Build history of the part. All positions in model axes, mm. A direction names the side the tool comes from. Give positions to 0.01 mm unless a question says otherwise; leave off trailing zeros. Order: outer loops, then holes, each group sorted by start corner. A loop starts at its lowest first (then second) coordinate and runs counter-clockwise, first axis right, second up. Notation, with made-up numbers: (23.5, -37.5) - (47.5, -37.5) arc R10 ccw to (47.5, -26.5) - close; hole circle Ø6 at (31, 3.25). An arc over 180 degrees is marked (long way). Answer in a Markdown table with one row per item.
```python
from build123d import *

# Parameters (mm, degrees)
F0_W     = 76.2
F0_H     = 76.2
F1_DEPTH = 76.2
F2_W     = 25.4
F2_H     = 25.4
F3_DEPTH = 12.7
F5_D     = 25.4
F6_R     = 15.048086
F7_DEPTH = 12.7


with BuildPart() as f1:
    # F0 (on Front) → F1 (new body)
    with BuildSketch(Plane.XZ):
        with Locations((5.308721, 14.755955)):
            Rectangle(F0_W, F0_H)
    extrude(amount=F1_DEPTH)

    # F2 (on face) → F3 (join)
    with BuildSketch(Plane.XZ.offset(76.2)):
        with Locations((5.308721, 14.755955)):
            Rectangle(F2_W, F2_H)
    extrude(amount=F3_DEPTH)

    # F5 (through all)
    with Locations(Plane.XY.offset(52.855955)):
        with Locations((0, -38.1)):
            Hole(F5_D / 2)

    # F6 (on face) → F7 (join)
    with BuildSketch(Plane.YZ.offset(43.408721)):
        with Locations((-40.448086, 17.104041)):
            Circle(F6_R)
    extrude(amount=F7_DEPTH)


solid = f1.part
```
1. Drop flat-ended pins along their axis: P1, Ø6.5, axis at x = 6.5, y = -81.5, coming from the +Z side; P2, Ø10, axis at y = -85, z = 10.5, coming from the +X side; P3, Ø6, axis at x = 40, z = 18.5, coming from the -Y side. Give the stop position or say it passes through.
Check result:
| item | result |
|---|---|
| P1 | stops at z = 27.46 |
| P2 | stops at x = 18.01 |
| P3 | stops at y = -76.2 |
2. Cut at B-B on y = -38.1. Write the cut outline in (x, z), and give its area (3 significant figures).
Check result:
| item | result |
|---|---|
| outline | (-32.79, -23.34) - (-12.7, -23.34) - (-12.7, 52.86) - (-32.79, 52.86) - close; (12.7, -23.34) - (43.41, -23.34) - (43.41, 2.24) - (56.11, 2.24) - (56.11, 31.97) - (43.41, 31.97) - (43.41, 52.86) - (12.7, 52.86) - close |
| area | 4,250 mm² |
3. Probe line 1 (Y direction, x = 0, z = 7); line 2 (Y direction, x = 0, z = -6); line 3 (X direction, y = -38, z = -4). List the from-to ranges inside material, lowest first.
Check result:
| item | result |
|---|---|
| line 1 | y = -88.9 to -50.8, -25.4 to 0 |
| line 2 | y = -76.2 to -50.8, -25.4 to 0 |
| line 3 | x = -32.79 to -12.7, 12.7 to 43.41 |
4. Which spindle directions (+Z, -Z, +X, -X, +Y, -Y) get a long thin tool onto all of the face, cutting with end or side? Do faces 4 (the face through (5, -82, 27.456)), 5 (the face through (-7.391, -82, 15)), 6 (the face through (43.409, -29, 6)), 7 (the face through (5, -82, 2.056)). Say none if no direction does.
Check result:
| item | result |
|---|---|
| face 4 | +Z, +X, -X, -Y |
| face 5 | +Z, -Z, -X, -Y |
| face 6 | +X |
| face 7 | -Z, +X, -X, -Y |
5. Cut at D-D on x = 36. Write the cut outline in (y, z), and give its area (3 significant figures).
Check result:
| item | result |
|---|---|
| outline | (-76.2, -23.34) - (0, -23.34) - (0, 52.86) - (-76.2, 52.86) - close |
| area | 5,810 mm² |
6. Two-plate mould, pull along Y, no slides. Class faces 1 (the face through (-32.791, -38, 14)), 2 (the face through (49.67, -55.48, 17.77)), 3 (the face through (2.75, -50.5, 14.22)): +Y half, -Y half, draft (parallel to the pull), parting line (faces both ways), or undercut.
Check result:
| item | result |
|---|---|
| face 1 | draft |
| face 2 | parting line |
| face 3 | undercut |
7. Cut at A-A on x = 0. Write the cut outline in (y, z).
Check result:
| item | result |
|---|---|
| outline | (-88.9, 2.06) - (-76.2, 2.06) - (-76.2, -23.34) - (-50.8, -23.34) - (-50.8, 52.86) - (-76.2, 52.86) - (-76.2, 27.46) - (-88.9, 27.46) - close; (-25.4, -23.34) - (0, -23.34) - (0, 52.86) - (-25.4, 52.86) - close |
8. Cut at C-C on z = 13.5. Write the cut outline in (x, y).
Check result:
| item | result |
|---|---|
| outline | (-32.79, -76.2) - (-7.39, -76.2) - (-7.39, -88.9) - (18.01, -88.9) - (18.01, -76.2) - (43.41, -76.2) - (43.41, -55.06) - (56.11, -55.06) - (56.11, -25.84) - (43.41, -25.84) - (43.41, 0) - (-32.79, 0) - close; hole circle Ø25.4 at (0, -38.1) |
